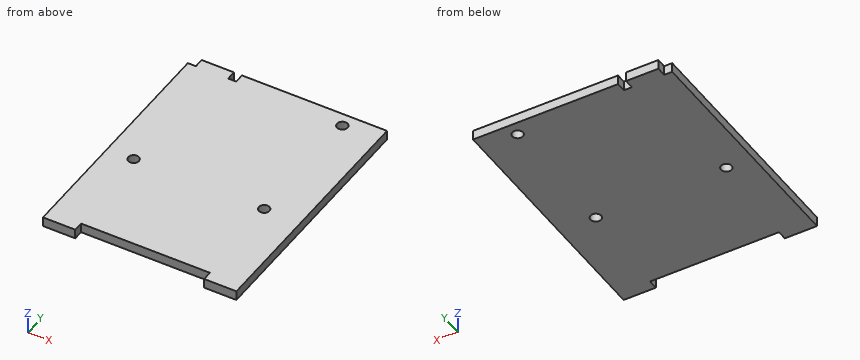
from build123d import *

# Parameters (mm, degrees)
SKETCH1_W              = 60
SKETCH1_H              = 75
MAINBODY_DEPTH         = 1.5
SHAFT_HOLES_DEPTH      = 110.668819634
SHAFT_HOLES_DEPTH_BACK = 110.668819634
SKETCH3_R              = 1.65
SKETCH4_W              = 10
SKETCH4_H              = 3
BASETABS_DEPTH         = 1.5
SKETCH5_W              = 2.5
SKETCH5_H              = 3
CUT_EXTRUDE2_DEPTH     = 110.69958979


with BuildPart() as part:
    # Sketch1 → MainBody (new, symmetric)
    with BuildSketch(Plane.XY):
        with Locations((50, 37.5)):
            Rectangle(SKETCH1_W, SKETCH1_H)
    extrude(amount=MAINBODY_DEPTH, both=True)

    # Sketch3 → Shaft Holes (cut, two sides: drawn at the far end of the back side and taken through both)
    with BuildSketch(Plane.XY.offset(-SHAFT_HOLES_DEPTH_BACK)):
        with Locations((28.190778624, 30.2606043)):
            Circle(SKETCH3_R)
        with Locations((68.690778624, 30.2606043)):
            Circle(SKETCH3_R)
        with Locations((68.690778624, 70.7606043)):
            Circle(SKETCH3_R)
    extrude(amount=SHAFT_HOLES_DEPTH + SHAFT_HOLES_DEPTH_BACK, mode=Mode.SUBTRACT)

    # Sketch4 → BaseTabs (add, symmetric)
    with BuildSketch(Plane.XY):
        with Locations((25, -1.5)):
            Rectangle(SKETCH4_W, SKETCH4_H)
        with Locations((75, -1.5)):
            Rectangle(SKETCH4_W, SKETCH4_H)
    extrude(amount=BASETABS_DEPTH, both=True)

    # Sketch5 → Cut-Extrude2 (cut, through all)
    with BuildSketch(Plane.XY.offset(1.5)):
        with Locations((21.25, 73.5)):
            Rectangle(SKETCH5_W, SKETCH5_H)
        with Locations((33.75, 73.5)):
            Rectangle(SKETCH5_W, SKETCH5_H)
    extrude(amount=-CUT_EXTRUDE2_DEPTH, mode=Mode.SUBTRACT)


solid = part.part
Input: part model. Units: mm. Frame: model coordinates. Round coordinates to 2 decimals unless told otherwise and drop trailing zeros. Order: outer loops, then holes, each group sorted by start corner. A loop starts at its lowest first (then second) coordinate and runs counter-clockwise, first axis right, second up. Notation, with made-up numbers: (-34, 23) - (24, 23) arc R9 ccw to (24, 32) - close; hole circle Ø4 at (9.25, 6.25). An arc over 180 degrees is marked (long way). Use a Markdown table: item, result.
1. Section A-A on z = 0.25. Return the cut outline in (x, y).
Evaluation:
| item | result |
|---|---|
| outline | (20, -3) - (30, -3) - (30, 0) - (70, 0) - (70, -3) - (80, -3) - (80, 75) - (35, 75) - (35, 72) - (32.5, 72) - (32.5, 75) - (22.5, 75) - (22.5, 72) - (20, 72) - close; hole circle Ø3.3 at (28.19, 30.26); hole circle Ø3.3 at (68.69, 30.26); hole circle Ø3.3 at (68.69, 70.76) |
2. Section B-B on x = 60.5. Return the cut outline in (y, z), then the cut area to 3 significant figures.
Evaluation:
| item | result |
|---|---|
| outline | (0, -1.5) - (75, -1.5) - (75, 1.5) - (0, 1.5) - close |
| area | 225 mm^2 |
3. First-contact query: pin 1 (1.2 mm diameter, centred on x = 21, z = -0.5, fed in from +Y). Flat tip, straight axial feed; report the tip coordinate or a pass-through.
Evaluation:
| item | result |
|---|---|
| pin 1 | y = 72 |
4. Material intervals for probe 1 along Y at (x, z) = (68, -0.25); probe 2 along Y at (x, z) = (67.5, -0.45); probe 3 along Y at (x, z) = (61, 0.4), sorted ascending.
Evaluation:
| item | result |
|---|---|
| probe 1 | 0 to 28.76, 31.76 to 69.26, 72.26 to 75 |
| probe 2 | 0 to 29.12, 31.4 to 69.62, 71.9 to 75 |
| probe 3 | 0 to 75 |
